from build123d import *

# Parameters (mm, degrees)
SKETCH2_R           = 50
BOSS_EXTRUDE1_DEPTH = 10
BOSS_EXTRUDE2_START = 10
BOSS_EXTRUDE2_DEPTH = 10
BOSS_EXTRUDE3_DEPTH = 10


with BuildPart() as part:
    # Sketch2 → Boss-Extrude1 (new body)
    with BuildSketch(Plane.XY):
        Circle(SKETCH2_R)
    extrude(amount=BOSS_EXTRUDE1_DEPTH)

    # Sketch3 → Boss-Extrude2 (add)
    with BuildSketch(Plane(origin=(0, 0, 0), x_dir=(-1, 0, 0), z_dir=(0, 0, -1)).offset(BOSS_EXTRUDE2_START)):
        with BuildLine():
            Line((-49.638694584, 6), (49.638694584, 6))
            ThreePointArc((49.638694584, 6), (50, 0), (49.638694584, -6))
            Line((49.638694584, -6), (-49.638694584, -6))
            ThreePointArc((-49.638694584, -6), (-50, 0), (-49.638694584, 6))
        make_face()
    extrude(amount=-BOSS_EXTRUDE2_DEPTH)

    # Sketch5 → Boss-Extrude3 (add)
    with BuildSketch(Plane.XY.offset(10)):
        with BuildLine():
            Line((-6, 49.638694584), (-6, -49.638694584))
            ThreePointArc((-6, -49.638694584), (0, -50), (6, -49.638694584))
            Line((6, -49.638694584), (6, 49.638694584))
            ThreePointArc((6, 49.638694584), (0, 50), (-6, 49.638694584))
        make_face()
    extrude(amount=BOSS_EXTRUDE3_DEPTH)


solid = part.part
Source: CAD feature listing. Evaluate the final solid. Frame: model axes, mm. A direction names the side the tool comes from. Coordinates: 2 decimals unless noted, no trailing zeros. Loops run counter-clockwise (first coordinate to the right, second up) from the corner with the lowest first, then second, coordinate; pieces in that order, holes last. Notation, with made-up numbers: (18.25, 5) - (43.25, 5) arc R20 cw to (43.25, 20) - close; hole circle Ø7 at (-32, 25). An arc over 180 degrees is marked (long way). Return JSON: item names as keys, results as strings.
Q1. Section D-D, the plane x = 29.5. Return loops of the section in (y, z).
Results:
{"outline": "(-40.37, 0) - (-6, 0) - (-6, -10) - (6, -10) - (6, 0) - (40.37, 0) - (40.37, 10) - (-40.37, 10) - close"}
Q2. Section C-C, the plane z = -1.5. Return loops of the section in (x, y), plus the area to 3 significant figures.
Results:
{"outline": "(-49.64, -6) - (49.64, -6) arc R50 ccw to (49.64, 6) - (-49.64, 6) arc R50 ccw to start", "area": "1,200 mm2"}
Q3. Contact query for flat-ended pins moving along their axis: P1, Ø3, axis at y = -30.5, z = 7, coming from the +X side; P2, Ø3, axis at x = -29.5, z = -6.5, coming from the +Y side; P3, Ø3, axis at x = -11.5, z = 13, coming from the +Y side; P4, Ø12, axis at x = 23, z = -1.5, coming from the -Y side. Output: stop coordinate, or through.
Results:
{"P1": "x = 40.73", "P2": "y = 6", "P3": "through", "P4": "y = -46.95"}
Q4. Material intervals for line 1 along X through (y, z) = (-44, 10.75); line 2 along Z through (x, y) = (-17, -18), sorted ascending.
Results:
{"line 1": "-6 to 6", "line 2": "0 to 10"}
Q5. Section A-A, the plane x = 0. Return loops of the section in (y, z).
Results:
{"outline": "(-50, 0) - (-6, 0) - (-6, -10) - (6, -10) - (6, 0) - (50, 0) - (50, 20) - (-50, 20) - close"}
Q6. Access query for faces 1 (the flat face through (-1, -6, -5)), 2 (the flat face through (-6, 1, 15)), 3 (the flat face through (23, 1, 10)). Directions: +Z, -Z, +X, -X, +Y, -Y. A direction counts if a zero-diameter tool reaches every point of the face in a straight line with its end or side. Return the directions, or none.
Results:
{"face 1": "-Z, +X, -X, -Y", "face 2": "+Z, -X, +Y, -Y", "face 3": "+Z, +X, +Y, -Y"}
Q7. Section B-B, the plane y = 0. Return loops of the section in (x, z), plus the area to 3 significant figures.
Results:
{"outline": "(-50, -10) - (50, -10) - (50, 10) - (6, 10) - (6, 20) - (-6, 20) - (-6, 10) - (-50, 10) - close", "area": "2,120 mm2"}
